from build123d import *

# Parameters (mm, degrees)
SKETCH1_W           = 24.303155339
SKETCH1_H           = 12.7
BOSS_EXTRUDE1_DEPTH = 12.7
SKETCH2_R           = 1.75
CUT_EXTRUDE1_DEPTH  = 14.224
SKETCH3_R           = 1.27
CUT_EXTRUDE2_DEPTH  = 31.219585693


with BuildPart() as part:
    # Sketch1 → Boss-Extrude1 (new body)
    with BuildSketch(Plane(origin=(0, 0, 0), x_dir=(1, 0, 0), z_dir=(0, 1, 0))):
        with Locations((12.151577669, 6.35)):
            Rectangle(SKETCH1_W, SKETCH1_H)
    extrude(amount=BOSS_EXTRUDE1_DEPTH)

    # Sketch2 → Cut-Extrude1 (cut)
    with BuildSketch(Plane.ZY):
        with Locations((-6.362201195, 6.35)):
            Circle(SKETCH2_R)
    extrude(amount=-CUT_EXTRUDE1_DEPTH, mode=Mode.SUBTRACT)

    # Sketch3 → Cut-Extrude2 (cut, through all)
    with BuildSketch(Plane(origin=(0, 0, 0), x_dir=(1, 0, 0), z_dir=(0, 1, 0))):
        with Locations(Location((17.953155339, 6.35, 0), (0, 0, 270))):
            Circle(SKETCH3_R)
    extrude(amount=CUT_EXTRUDE2_DEPTH, mode=Mode.SUBTRACT)


solid = part.part
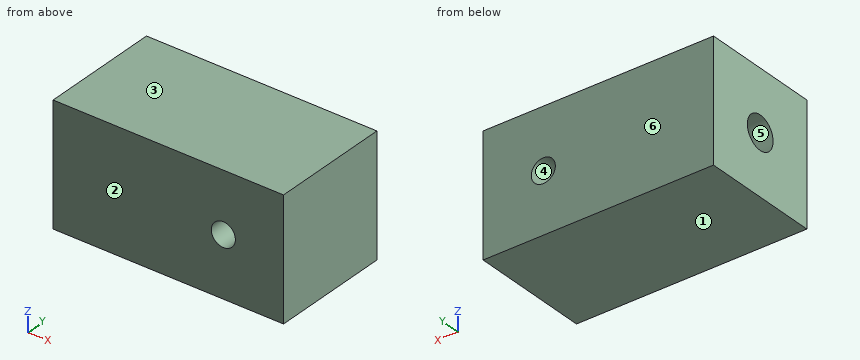
Source: CAD feature listing. Evaluate the final solid. Frame: model axes, mm. Face numbers are marked on the shaded views. A direction names the side the tool comes from. Round coordinates to 2 decimals unless told otherwise and drop trailing zeros. Loops run counter-clockwise (first coordinate to the right, second up) from the corner with the lowest first, then second, coordinate; pieces in that order, holes last. Notation, with made-up numbers: (6, 61.5) -> (28, 61.5) arc R23 cw to (28, 92.5) -> close; hole circle Ø9 at (65, 12). An arc over 180 degrees is marked (long way). Answer as a JSON object with one key per item and string values. Group by question number.
Q1. Section query B-B (x = 3.25). Output: boundary loops of the cut face in (y, z), plus the area to 3 significant figures.
Q2. Section query D-D (y = 5.5). Output: boundary loops of the cut face in (x, z), plus the area to 3 significant figures.
Q3. Access query for the marked faces 5 and 6. Directions: +Z, -Z, +X, -X, +Y, -Y. A direction counts if a zero-diameter tool reaches every point of the face in a straight line with its end or side. Return the directions, or none.
Q4. Section query C-C (x = 18.5). Output: boundary loops of the cut face in (y, z).
Q5. Mould query, pull axis Z, two halves, no side actions, for the marked faces 1, 2, 3 and 4. Classes: pulls with the +Z half, pulls with the -Z half, needs draft (parallel to the pull), parting line crosses it, or undercut.
Q6. Section query A-A (z = -7). Output: boundary loops of the cut face in (x, y), plus the area to 3 significant figures.
Q7. Ray query, line 1 (Y direction, x = 6, z = -6.5); line 2 (X direction, y = 5, z = -6.35); line 3 (X direction, y = 3.5, z = -6.35). Return the intervals inside material, ascending. Write a range as from..to.
Completed:
{
 "1": {"outline": "(0, -12.7) -> (12.7, -12.7) -> (12.7, 0) -> (0, 0) -> close; hole circle Ø3.5 at (6.35, -6.36)", "area": "152 mm²"},
 "2": {"outline": "(0, -12.7) -> (24.3, -12.7) -> (24.3, 0) -> (0, 0) -> (0, -4.83) -> (14.22, -4.83) -> (14.22, -7.89) -> (0, -7.89) -> close; hole circle Ø2.54 at (17.95, -6.35)", "area": "260 mm²"},
 "3": {"face 5": "-X", "face 6": "+Z, -Z, +X, -X, +Y"},
 "4": {"outline": "(0, -12.7) -> (12.7, -12.7) -> (12.7, -7.5) -> (0, -7.5) -> close; (0, -5.2) -> (12.7, -5.2) -> (12.7, 0) -> (0, 0) -> close"},
 "5": {"face 1": "pulls with the -Z half", "face 2": "needs draft", "face 3": "pulls with the +Z half", "face 4": "undercut"},
 "6": {"outline": "(0, 0) -> (16.86, 0) -> (16.86, 12.7) -> (0, 12.7) -> (0, 7.98) -> (14.22, 7.98) -> (14.22, 4.72) -> (0, 4.72) -> close; (19.04, 0) -> (24.3, 0) -> (24.3, 12.7) -> (19.04, 12.7) -> close", "area": "235 mm²"},
 "7": {"line 1": "0..4.61, 8.09..12.7", "line 2": "14.22..16.68, 19.22..24.3", "line 3": "0..16.68, 19.22..24.3"}
}
